Here's how the part is built. I have some questions about the finished solid (model axes, mm). Round coordinates to 2 decimals unless told otherwise and drop trailing zeros. Loops run counter-clockwise (first coordinate to the right, second up) from the corner with the lowest first, then second, coordinate; pieces in that order, holes last. Notation, with made-up numbers: (2.25, -24) -> (49.25, -24) arc R19 ccw to (49.25, 9) -> close; hole circle Ø11 at (12.5, 58.5). An arc over 180 degrees is marked (long way). Use one line per item in the form item = value. Start each with the question number.
Item 1: Thinking about a two-plate mould opening in X: for faces 1 (the face through (-123.18, 3.13, 123.38)), 2 (the face through (42.397, 3.131, -13.352)), 3 (the face through (2, 6.35, 55)), which applies, released by +X, released by -X, zero draft, split by the parting line, or undercut?
Item 2: If we section it at D-D (y = 1.5): Write out the boundary of the cut face in (x, z) (3 decimals).
Item 3: If we section it at C-C (z = 19.5): Write out the boundary of the cut face in (x, y).
Item 4: I'm going to push flat-ended pins straight in: pin 1 Ø2 at (x, z) = (-81.5, -67.5) entering from -Y; pin 2 Ø10 at (x, z) = (86.26, 74.99) entering from -Y; pin 3 Ø3 at (x, y) = (78.5, 5) entering from -Z. Where does each tip first touch, or does it pass through?
Item 5: If we section it at B-B (z = 107.95): Write out the boundary of the cut face in (x, y) (3 decimals), then the cut area to 3 significant figures.
Item 6: If I drill on L1, parallel to X at y = 3.5, z = 107.95 (3 decimals); L2, parallel to Z at x = 19.5, y = 1; L3, parallel to X at y = 3.25, z = 0, over which ranges is the centre line in solid material (lowest first)? Write a range as [from, to].
Item 7: If we section it at A-A (x = 0): Write out the boundary of the cut face in (y, z).
```python
from build123d import *

# Parameters (mm, degrees)
SKETCH1_R           = 44.45
SKETCH1_R_2         = 6.35
SKETCH1_R_3         = 3.175
BOSS_EXTRUDE1_DEPTH = 6.35
SKETCH6_R           = 14.2875
SKETCH6_R_2         = 11.176
CUT_EXTRUDE1_DEPTH  = 28.448


with BuildPart() as part:
    # Sketch1 → Boss-Extrude1 (new body)
    with BuildSketch(Plane(origin=(0, 0, 0), x_dir=(1, 0, 0), z_dir=(0, 1, 0))):
        with BuildLine():
            Line((127, 0), (127, -114.3))
            ThreePointArc((127, -114.3), (123.280256121, -123.280256121), (114.3, -127))
            Line((114.3, -127), (-114.3, -127))
            ThreePointArc((-114.3, -127), (-123.280256121, -123.280256121), (-127, -114.3))
            Line((-127, -114.3), (-127, 0))
            ThreePointArc((-127, 0), (0, 127), (127, 0))
        make_face()
        Circle(SKETCH1_R, mode=Mode.SUBTRACT)
        with Locations((-108.072773191, -37.212440054)):
            Circle(SKETCH1_R_2, mode=Mode.SUBTRACT)
        with Locations((21.809468172, 112.199987068)):
            Circle(SKETCH1_R_2, mode=Mode.SUBTRACT)
        with Locations((86.263305019, -74.987547014)):
            Circle(SKETCH1_R_2, mode=Mode.SUBTRACT)
        with Locations((-76.2, -107.95)):
            Circle(SKETCH1_R_3, mode=Mode.SUBTRACT)
        with Locations((76.2, -107.95)):
            Circle(SKETCH1_R_3, mode=Mode.SUBTRACT)
    extrude(amount=BOSS_EXTRUDE1_DEPTH)

    # Sketch6 → Cut-Extrude1 (cut)
    with BuildSketch(Plane(origin=(0, 0, 0), x_dir=(1, 0, 0), z_dir=(0, 1, 0))):
        with Locations((174.752, 0)):
            Circle(SKETCH6_R)
        with Locations((174.752, 0)):
            Circle(SKETCH6_R_2, mode=Mode.SUBTRACT)
    extrude(amount=CUT_EXTRUDE1_DEPTH, mode=Mode.SUBTRACT)


solid = part.part
```
Values found:
q1.face_1 = released by -X
q1.face_2 = undercut
q1.face_3 = zero draft
q2.outline = (-127, 0) arc R127 ccw to (127, 0) -> (127, 114.3) arc R12.7 ccw to (114.3, 127) -> (-114.3, 127) arc R12.7 ccw to (-127, 114.3) -> close; hole circle Ø12.7 at (-108.073, 37.212); hole circle Ø6.35 at (-76.2, 107.95); hole circle Ø88.9 at (0, 0); hole circle Ø12.7 at (21.809, -112.2); hole circle Ø6.35 at (76.2, 107.95); hole circle Ø12.7 at (86.263, 74.988)
q3.outline = (-127, 0) -> (-39.94, 0) -> (-39.94, 6.35) -> (-127, 6.35) -> close; (39.94, 0) -> (127, 0) -> (127, 6.35) -> (39.94, 6.35) -> close
q4.pin_1 = 0
q4.pin_2 = through
q4.pin_3 = -101
q5.outline = (-127, 0) -> (-79.375, 0) -> (-79.375, 6.35) -> (-127, 6.35) -> close; (-73.025, 0) -> (73.025, 0) -> (73.025, 6.35) -> (-73.025, 6.35) -> close; (79.375, 0) -> (127, 0) -> (127, 6.35) -> (79.375, 6.35) -> close
q5.area = 1,530 mm2
q6.L1 = [-127, -79.375], [-73.025, 73.025], [79.375, 127]
q6.L2 = [-125.49, -118.12], [-106.28, -39.94], [39.94, 127]
q6.L3 = [-127, -44.45], [44.45, 127]
q7.outline = (0, -127) -> (6.35, -127) -> (6.35, -44.45) -> (0, -44.45) -> close; (0, 44.45) -> (6.35, 44.45) -> (6.35, 127) -> (0, 127) -> close
